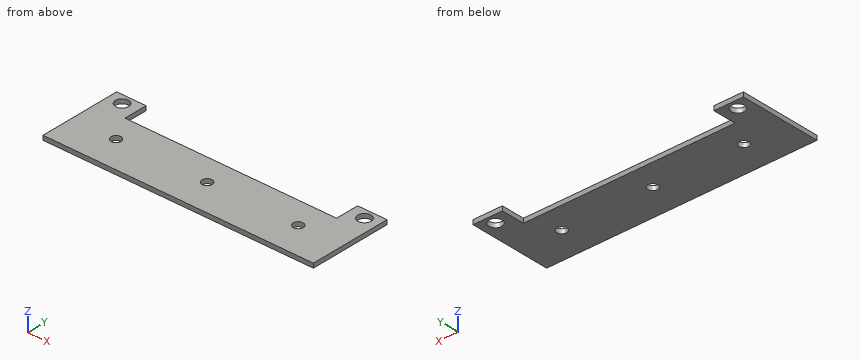
from build123d import *

# Parameters (mm, degrees)
PAD_DEPTH     = 1.5
SKETCH001_R   = 1.7
HOLE_DEPTH    = 25
SKETCH002_R   = 2.25
HOLE001_DEPTH = 25


with BuildPart() as part:
    # Sketch → Pad (new body)
    with BuildSketch(Plane.XY):
        Polygon((-36, 14), (-46, 14), (-46, -14), (46, -14), (46, 14), (36, 14), (36, 6), (-36, 6), align=None)
    extrude(amount=PAD_DEPTH)

    # Sketch001 (on Face10 of Pad) → Hole (cut)
    with BuildSketch(Plane.XY.offset(1.5)):
        with Locations((31, -3)):
            Circle(SKETCH001_R)
        with Locations((0, -3)):
            Circle(SKETCH001_R)
        with Locations((-31, -3)):
            Circle(SKETCH001_R)
    extrude(amount=-HOLE_DEPTH, mode=Mode.SUBTRACT)

    # Sketch002 (on Face5 of Hole) → Hole001 (cut)
    with BuildSketch(Plane.XY.offset(1.5)):
        with Locations((-41.25, 10.75)):
            Circle(SKETCH002_R)
        with Locations((41.25, 10.75)):
            Circle(SKETCH002_R)
    extrude(amount=-HOLE001_DEPTH, mode=Mode.SUBTRACT)


solid = part.part
Can you work these out from the model? Positions are in its coordinate system, mm. Give positions to 0.01 mm unless a question says otherwise; leave off trailing zeros. Loops run counter-clockwise (first coordinate to the right, second up) from the corner with the lowest first, then second, coordinate; pieces in that order, holes last. Notation, with made-up numbers: (-13, 20.25) - (2, 20.25) arc R19 ccw to (2, 40.25) - close; hole circle Ø5 at (38, 39.5). An arc over 180 degrees is marked (long way). Return JSON: item names as keys, results as strings.
1. I want a section at C-C on z = 1.15. Please give me the cut outline in (x, y).
Output values:
{"outline": "(-46, -14) - (46, -14) - (46, 14) - (36, 14) - (36, 6) - (-36, 6) - (-36, 14) - (-46, 14) - close; hole circle Ø4.5 at (-41.25, 10.75); hole circle Ø3.4 at (-31, -3); hole circle Ø3.4 at (0, -3); hole circle Ø3.4 at (31, -3); hole circle Ø4.5 at (41.25, 10.75)"}
2. I want a section at D-D on x = 31.5. Please give me the cut outline in (y, z), and give its area (3 significant figures).
Output values:
{"outline": "(-14, 0) - (-4.62, 0) - (-4.62, 1.5) - (-14, 1.5) - close; (-1.38, 0) - (6, 0) - (6, 1.5) - (-1.38, 1.5) - close", "area": "25.1 mm²"}
3. I want a section at A-A on y = -3. Please give me the cut outline in (x, z).
Output values:
{"outline": "(-46, 0) - (-32.7, 0) - (-32.7, 1.5) - (-46, 1.5) - close; (-29.3, 0) - (-1.7, 0) - (-1.7, 1.5) - (-29.3, 1.5) - close; (1.7, 0) - (29.3, 0) - (29.3, 1.5) - (1.7, 1.5) - close; (32.7, 0) - (46, 0) - (46, 1.5) - (32.7, 1.5) - close"}
4. If I drill on line 1 (Y direction, x = 31, z = 1); line 2 (Y direction, x = -7, z = 0.45); line 3 (X direction, y = 8.75, z = 1.25), over which ranges is the centre line in solid material (lowest first)?
Output values:
{"line 1": "y = -14 to -4.7, -1.3 to 6", "line 2": "y = -14 to 6", "line 3": "x = -46 to -42.28, -40.22 to -36, 36 to 40.22, 42.28 to 46"}
5. I want a section at B-B on x = 41.25. Please give me the cut outline in (y, z).
Output values:
{"outline": "(-14, 0) - (8.5, 0) - (8.5, 1.5) - (-14, 1.5) - close; (13, 0) - (14, 0) - (14, 1.5) - (13, 1.5) - close"}
6. I'm going to push a flat-ended pin straight in: pin 1 Ø4 at (x, y) = (-41.25, 10.75) entering from +Z. Where does the tip first touch, or does it pass through?
Output values:
{"pin 1": "passes through"}
